Part model, mm, in its own coordinate system. A direction names the side the tool comes from. Give positions to 0.01 mm unless a question says otherwise; leave off trailing zeros. Write each loop counter-clockwise with the first axis right and the second up, starting at its lowest first coordinate (ties: lowest second). Pieces come first, ordered by that corner, then holes. Notation, with made-up numbers: (89, -12) - (120, -12) arc R18 cw to (120, 9) - close; hole circle Ø9 at (75, -29). An arc over 180 degrees is marked (long way). Answer in a Markdown table with one row per item. Add a question column.
1. Drop a flat-ended pin along its axis: pin 1 Ø1.5 at (y, z) = (31, 7) entering from -X. Give the stop position or say it passes through.
2. Probe line 1 along Y through (x, z) = (37, 7.5); line 2 along X through (y, z) = (13, 6.5); line 3 along Y through (x, z) = (17.5, 3). List the from-to ranges inside material, lowest first.
3. Band-saw the part on A-A on x = 15.5. Write the cut outline in (y, z).
4. Band-saw the part on C-C on z = 5.75. State how many separate pieces and enclosed holes the cut face has, plus the area to 3 significant figures.
5. Band-saw the part on B-B on y = 26.5. Write the cut outline in (x, z), plus the area to 3 significant figures.
6. Pull direction Y, two halves, no side cores. Call faces 1 (the cylindrical face through (72, 33, 4)), 2 (the flat face through (44, 18, 0)), 3 (the cylindrical face through (61.1, 14.1, 4.5)): released by +Y, released by -Y, zero draft, split by the parting line, or undercut.
7. Which spindle directions (+Z, -Z, +X, -X, +Y, -Y) get a long thin tool onto all of the face, cutting with end or side? Do faces 4 (the cylindrical face through (61, 20, 1)), 5 (the cylindrical face through (14.79, 5.297, 3.944)). Say none if no direction does.
8. Band-saw the part on D-D on x = 42. Write the cut outline in (y, z), plus the area to 3 significant figures.
```python
from build123d import *

# Parameters (mm, degrees)
F0_R     = 12.5
F1_DEPTH = 8


with BuildPart() as f1:
    # F0 (on Top) → F1 (new body)
    with BuildSketch(Plane.XY):
        with BuildLine():
            ThreePointArc((0, 17.5), (5.125631, 5.125631), (17.5, 0))
            Line((17.5, 0), (68, 0))
            ThreePointArc((68, 0), (71.535534, 1.464466), (73, 5))
            Line((73, 5), (73, 30))
            ThreePointArc((73, 30), (71.535534, 33.535534), (68, 35))
            Line((68, 35), (17.5, 35))
            ThreePointArc((17.5, 35), (5.125631, 29.874369), (0, 17.5))
        make_face()
        with Locations((17.5, 17.5)):
            Circle(F0_R, mode=Mode.SUBTRACT)
    extrude(amount=F1_DEPTH)

    # F2 (on face) → F3 (revolve, cut)
    with BuildSketch(Plane.XY.offset(8)):
        Polygon((42, 19), (42, 9), (45.5, 9), (45.5, 19), (49, 19), (49, 21.2), (48, 21.2), (48, 25.7), (42, 25.7), (42, 21.2), align=None)
    revolve(axis=Axis((42, 14, 8), (0, 1, 0)), mode=Mode.SUBTRACT)

    # F2 (on face) → F4 (revolve, cut)
    with BuildSketch(Plane.XY.offset(8)):
        Polygon((61, 19), (61, 9), (64.5, 9), (64.5, 19), (68, 19), (68, 21.2), (67, 21.2), (67, 25.7), (61, 25.7), (61, 21.2), align=None)
    revolve(axis=Axis((61, 14, 8), (0, 1, 0)), mode=Mode.SUBTRACT)


solid = f1.part
```
Values:
| question | item | result |
|---|---|---|
| 1 | pin 1 | stops at x = 5.51 |
| 2 | line 1 | y = 0 to 19, 25.7 to 35 |
| 2 | line 2 | x = 0.59 to 5.84, 29.16 to 38.84, 45.16 to 57.84, 64.16 to 73 |
| 2 | line 3 | y = 0 to 5, 30 to 35 |
| 3 | outline | (0.11, 0) - (5.16, 0) - (5.16, 8) - (0.11, 8) - close; (29.84, 0) - (34.89, 0) - (34.89, 8) - (29.84, 8) - close |
| 4 | separate pieces | 1 |
| 4 | enclosed holes | 3 |
| 4 | area | 1,660 mm² |
| 5 | outline | (2.49, 0) - (8.83, 0) - (8.83, 8) - (2.49, 8) - close; (26.17, 0) - (73, 0) - (73, 8) - (26.17, 8) - close |
| 5 | area | 425 mm² |
| 6 | face 1 | released by +Y |
| 6 | face 2 | zero draft |
| 6 | face 3 | undercut |
| 7 | face 4 | +Z |
| 7 | face 5 | +Z, -Z |
| 8 | outline | (0, 0) - (35, 0) - (35, 8) - (25.7, 8) - (25.7, 2) - (21.2, 2) - (21.2, 1) - (19, 1) - (19, 4.5) - (9, 4.5) - (9, 8) - (0, 8) - close |
| 8 | area | 203 mm² |
